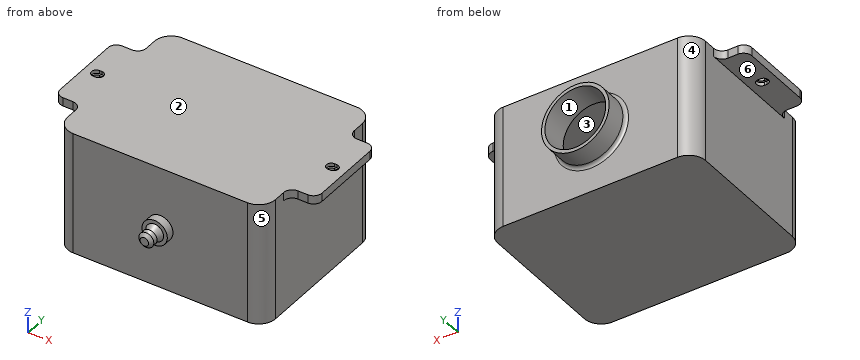
```python
from build123d import *

# Parameters (mm, degrees)
SKETCH1_W           = 156.21
SKETCH1_H           = 139.874625
BOSS_EXTRUDE1_DEPTH = 91.948
BOSS_EXTRUDE2_DEPTH = 6.35
SKETCH4_R           = 25.4
BOSS_EXTRUDE3_DEPTH = 17.859375
SKETCH5_W           = 156.21
SKETCH5_H           = 17.859375
CUT_EXTRUDE2_DEPTH  = 254.874905946
FILLET2_R           = 12.7
SHELL3_START        = 2.54
SHELL3_DEPTH        = 86.868
SHELL3_START_2      = 88.138
SHELL3_2_DEPTH      = 1.27
SHELL3_START_3      = 137.334625
SHELL3_3_OUTLINE_R  = 22.86
SHELL3_3_DEPTH      = 20.399375
FILLET3_R           = 6.35
SKETCH9_W           = 1.7859375
SKETCH9_H           = 7.14375
CUT_EXTRUDE3_DEPTH  = 254.874905946
FILLET4_R           = 2.54


with BuildPart() as part:
    # Sketch1 → Boss-Extrude1 (new body)
    with BuildSketch(Plane.XY):
        with Locations((78.105, 69.9373125)):
            Rectangle(SKETCH1_W, SKETCH1_H)
    extrude(amount=BOSS_EXTRUDE1_DEPTH)

    # Sketch3 → Boss-Extrude2 (add)
    with BuildSketch(Plane.XY.offset(91.948)):
        with BuildLine():
            Line((0, 111.887), (-13.843, 111.887))
            ThreePointArc((-13.843, 111.887), (-18.333128061, 110.027128061), (-20.193, 105.537))
            Line((-20.193, 105.537), (-20.193, 52.197))
            ThreePointArc((-20.193, 52.197), (-18.333128061, 47.706871939), (-13.843, 45.847))
            Line((-13.843, 45.847), (0, 45.847))
            Line((0, 45.847), (0, 111.887))
        make_face()
        with BuildLine():
            Line((156.21, 111.887), (170.053, 111.887))
            ThreePointArc((170.053, 111.887), (174.543128061, 110.027128061), (176.403, 105.537))
            Line((176.403, 105.537), (176.403, 52.197))
            ThreePointArc((176.403, 52.197), (174.543128061, 47.706871939), (170.053, 45.847))
            Line((170.053, 45.847), (156.21, 45.847))
            Line((156.21, 45.847), (156.21, 111.887))
        make_face()
    extrude(amount=-BOSS_EXTRUDE2_DEPTH)

    # Sketch4 → Boss-Extrude3 (add)
    with BuildSketch(Plane(origin=(0, 139.874625, 0), x_dir=(1, 0, 0), z_dir=(0, 1, 0))):
        with Locations(Location((77.343, -45.974, 0), (0, 0, 270))):
            Circle(SKETCH4_R)
    extrude(amount=BOSS_EXTRUDE3_DEPTH)

    # Sketch5 → Cut-Extrude2 (cut, through all)
    with BuildSketch(Plane.XY.offset(91.948)):
        with Locations((78.105, 8.9296875)):
            Rectangle(SKETCH5_W, SKETCH5_H)
    extrude(amount=-CUT_EXTRUDE2_DEPTH, mode=Mode.SUBTRACT)

    # Sketch6 → Revolve1 (revolve)
    with BuildSketch(Plane(origin=(0, 0, 45.974), x_dir=(-1, 0, 0), z_dir=(0, 0, -1)), mode=Mode.PRIVATE) as revolve1_sk:
        Polygon((-78.105, 17.859375), (-78.105, 0), (-81.28, 0), (-83.732198932, 2.205295997), (-81.28, 2.205295997), (-83.732198932, 5.846722634), (-81.28, 5.846722634), (-84.791652888, 11.509375), (-87.63, 11.509375), (-87.63, 17.859375), align=None)
    revolve(revolve1_sk.sketch.rotate(Axis((78.105, 17.859375, 45.974), (0, -1, 0)), 90), axis=Axis((78.105, 17.859375, 45.974), (0, -1, 0)))

    # Fillet2
    fillet2_edges = [part.edges().sort_by_distance(p)[0] for p in [
        (0, 17.859375, 45.974),
        (156.21, 17.859375, 45.974),
        (0, 139.874625, 45.974),
        (156.21, 139.874625, 45.974),
    ]]
    fillet(fillet2_edges, radius=FILLET2_R)

    # Shell3: read off the stored shape, not the designer's step
    # Shell3 outline → Shell3 (cut)
    with BuildSketch(Plane.XY.offset(SHELL3_START)):
        with BuildLine():
            ThreePointArc((12.7, 137.334625), (5.515795103, 134.358829897), (2.54, 127.174625))
            Line((2.54, 127.174625), (2.54, 30.559375))
            ThreePointArc((2.54, 30.559375), (5.515795103, 23.375170103), (12.7, 20.399375))
            Line((12.7, 20.399375), (143.51, 20.399375))
            ThreePointArc((143.51, 20.399375), (150.694204897, 23.375170103), (153.67, 30.559375))
            Line((153.67, 30.559375), (153.67, 127.174625))
            ThreePointArc((153.67, 127.174625), (150.694204897, 134.358829897), (143.51, 137.334625))
            Line((143.51, 137.334625), (12.7, 137.334625))
        make_face()
    extrude(amount=SHELL3_DEPTH, mode=Mode.SUBTRACT)

    # Shell3 2 outline → Shell3 2 (cut)
    with BuildSketch(Plane.XY.offset(SHELL3_START_2)):
        with BuildLine():
            Line((2.54, 48.387), (2.54, 109.347))
            Line((2.54, 109.347), (-13.843, 109.347))
            ThreePointArc((-13.843, 109.347), (-16.537076836, 108.231076836), (-17.653, 105.537))
            Line((-17.653, 105.537), (-17.653, 52.197))
            ThreePointArc((-17.653, 52.197), (-16.537076836, 49.502923164), (-13.843, 48.387))
            Line((-13.843, 48.387), (2.54, 48.387))
        make_face()
        with BuildLine():
            Line((170.053, 109.347), (153.67, 109.347))
            Line((153.67, 109.347), (153.67, 48.387))
            Line((153.67, 48.387), (170.053, 48.387))
            ThreePointArc((170.053, 48.387), (172.747076836, 49.502923164), (173.863, 52.197))
            Line((173.863, 52.197), (173.863, 105.537))
            ThreePointArc((173.863, 105.537), (172.747076836, 108.231076836), (170.053, 109.347))
        make_face()
    extrude(amount=SHELL3_2_DEPTH, mode=Mode.SUBTRACT)

    # Shell3 3 outline → Shell3 3 (cut)
    with BuildSketch(Plane(origin=(0, 0, 0), x_dir=(1, 0, 0), z_dir=(0, 1, 0)).offset(SHELL3_START_3)):
        with Locations((77.343, -45.974)):
            Circle(SHELL3_3_OUTLINE_R)
    extrude(amount=SHELL3_3_DEPTH, mode=Mode.SUBTRACT)

    # Shell3 4 outline → Shell3 4 (revolve, cut)
    with BuildSketch(Plane(origin=(78.105, 0, 45.974), x_dir=(1, 0, 0), z_dir=(0, 0, 1))):
        Polygon((0, 20.399375), (0, 5.546418432), (5.273046986, 14.049375), (6.985, 14.049375), (6.985, 20.399375), align=None)
        Polygon((0.854475277, 3.306722634), (0, 3.306722634), (0, 2.037857783), align=None)
    revolve(axis=Axis((78.105, 0, 45.974), (0, 1, 0)), mode=Mode.SUBTRACT)

    # Fillet3
    fillet3_edges = [part.edges().sort_by_distance(p)[0] for p in [
        (0, 111.887, 88.773),
        (0, 45.847, 88.773),
        (156.21, 45.847, 88.773),
        (156.21, 111.887, 88.773),
    ]]
    fillet(fillet3_edges, radius=FILLET3_R)

    # Sketch9 → Cut-Extrude3 (cut, through all)
    with BuildSketch(Plane.XY.offset(91.948)):
        with BuildLine():
            Line((-10.98946875, 82.438875), (-10.98946875, 75.295125))
            ThreePointArc((-10.98946875, 75.295125), (-14.56134375, 78.867), (-10.98946875, 82.438875))
        make_face()
        with BuildLine():
            ThreePointArc((-9.20353125, 82.438875), (-5.63165625, 78.867), (-9.20353125, 75.295125))
            Line((-9.20353125, 75.295125), (-9.20353125, 82.438875))
        make_face()
        with Locations((-10.0965, 78.867)):
            Rectangle(SKETCH9_W, SKETCH9_H)
        with BuildLine():
            Line((165.41353125, 82.438875), (165.41353125, 75.295125))
            ThreePointArc((165.41353125, 75.295125), (161.84165625, 78.867), (165.41353125, 82.438875))
        make_face()
        with BuildLine():
            ThreePointArc((167.19946875, 82.438875), (170.77134375, 78.867), (167.19946875, 75.295125))
            Line((167.19946875, 75.295125), (167.19946875, 82.438875))
        make_face()
        with Locations((166.3065, 78.867)):
            Rectangle(SKETCH9_W, SKETCH9_H)
    extrude(amount=-CUT_EXTRUDE3_DEPTH, mode=Mode.SUBTRACT)

    # Fillet4
    fillet4_edges = [part.edges().sort_by_distance(p)[0] for p in [
        (77.343, 139.874625, 20.574),
    ]]
    fillet(fillet4_edges, radius=FILLET4_R)


solid = part.part
```
CAD build for the part. Positions are in the model's coordinates, mm. Face numbers are marked on the shaded views. A direction names the side the tool comes from. Round coordinates to 2 decimals unless told otherwise and drop trailing zeros. Order: outer loops, then holes, each group sorted by start corner. A loop starts at its lowest first (then second) coordinate and runs counter-clockwise, first axis right, second up.
Item 1: Saw through at B-B on x = 15.5. Write the cut outline in (y, z), then the cut area to 3 significant figures.
Item 2: Mould opens along X. For the marked faces 3, 4, 5 and 6 say: pulls with the +X half, pulls with the -X half, needs draft (parallel to the pull), parting line crosses it, or undercut.
Item 3: Pin check, flat tips, straight feed: pin 1 (6 mm diameter, centred on y = 82.5, z = 62.5, fed in from +X); pin 2 (1.9 mm diameter, centred on x = -8, z = 87.5, fed in from -Y); pin 3 (2 mm diameter, centred on x = 43, z = 26, fed in from +Y); pin 4 (22 mm diameter, centred on x = 162.5, y = 96, fed in from -Z). Stop position of each tip, or through.
Item 4: Saw through at A-A on y = 87. Write the cut outline in (x, z), then the cut area to 3 significant figures.
Item 5: Probe line 1 along Z through (x, y) = (125, 74.5); line 2 along X through (y, z) = (31, 61); line 3 along Y through (x, z) = (82, 8.5). List the from-to ranges inside material, lowest first.
Item 6: Tool access for the marked faces 1 and 2: list every direction of +Z, -Z, +X, -X, +Y, -Y with a clear straight run to the whole face (end or side of a thin tool).
Reported:
1. outline: (17.86, 0) - (139.87, 0) - (139.87, 91.95) - (17.86, 91.95) - close; hole (20.4, 2.54) - (137.33, 2.54) - (137.33, 89.41) - (20.4, 89.41) - close
1. area: 1,060 mm2
2. face 3: undercut
2. face 4: pulls with the -X half
2. face 5: pulls with the +X half
2. face 6: needs draft
3. pin 1: stops at x = 156.21
3. pin 2: stops at y = 45.85
3. pin 3: stops at y = 139.87
3. pin 4: stops at z = 0
4. outline: (-20.19, 85.6) - (0, 85.6) - (0, 0) - (156.21, 0) - (156.21, 85.6) - (176.4, 85.6) - (176.4, 91.95) - (-20.19, 91.95) - close; hole (-17.65, 88.14) - (2.54, 88.14) - (2.54, 2.54) - (153.67, 2.54) - (153.67, 88.14) - (173.86, 88.14) - (173.86, 89.41) - (-17.65, 89.41) - close
4. area: 1,440 mm2
5. line 1: z = 0 to 2.54, 89.41 to 91.95
5. line 2: x = 0 to 2.54, 153.67 to 156.21
5. line 3: y = 17.86 to 20.4, 137.33 to 139.87
6. face 1: +Y
6. face 2: +Z, +X, -X, +Y, -Y
